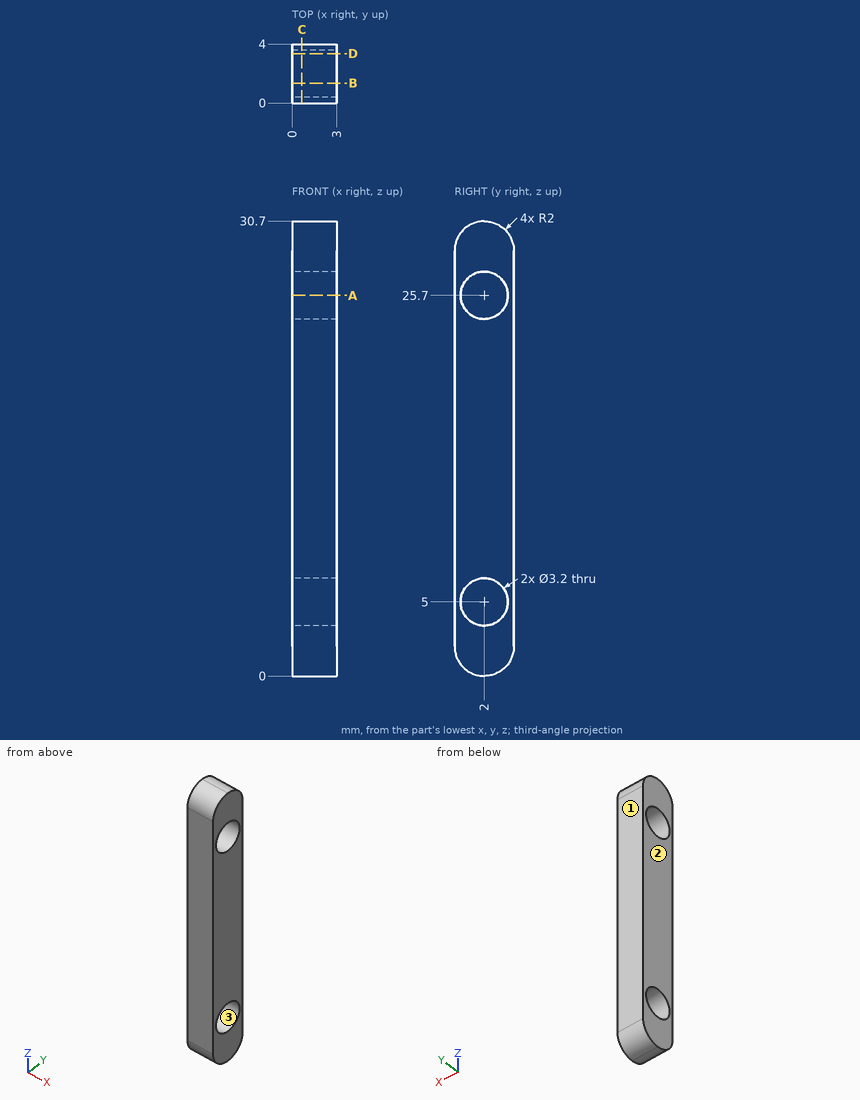
The figure shows three views and two pictorial views of one solid part (mm, origin at its lowest corner). Answer the questions. Round coordinates to 2 decimals unless told otherwise and drop trailing zeros. Write each loop counter-clockwise with the first axis right and the second up, starting at its lowest first coordinate (ties: lowest second). Pieces come first, ordered by that corner, then holes. Notation, with made-up numbers: (2, -2.5) -> (7, -2.5) arc R19 ccw to (7, 22.5) -> close; hole circle Ø1 at (51, 23). An arc over 180 degrees is marked (long way). Answer as a JSON object with one key per item and string values. Group by question number.
Q1. Section D-D (y = 3.35) is taken. Write down the section's boundary in (x, z) (1 decimal).
Q2. Section A-A (z = 25.7) is taken. Write down the section's boundary in (x, y).
Q3. Section C-C (x = 0.65) is taken. Count the separate pieces of the cut face and the enclosed holes in it, plus the area to 3 significant figures.
Q4. Straight lines are drawn through the part: line 1 along Z through (x, y) = (1.35, 2); line 2 along Y through (x, z) = (1.1, 25.7); line 3 along Z through (x, y) = (0.95, 2.95) (1 decimal). For each, find the intervals that lie inside material, in ascending order.
Q5. Section B-B (y = 1.35) is taken. Write down the section's boundary in (x, z).
Q6. Determine the mould class of the marked faces 1, 2 and 3 for opening direction Y: pulls with the +Y half, pulls with the -Y half, needs draft (parallel to the pull), parting line crosses it, or undercut.
Check values:
{
 "1": {"outline": "(0, 0.5) -> (3, 0.5) -> (3, 4.1) -> (0, 4.1) -> close; (0, 5.9) -> (3, 5.9) -> (3, 24.8) -> (0, 24.8) -> close; (0, 26.6) -> (3, 26.6) -> (3, 30.2) -> (0, 30.2) -> close"},
 "2": {"outline": "(0, 0) -> (3, 0) -> (3, 0.4) -> (0, 0.4) -> close; (0, 3.6) -> (3, 3.6) -> (3, 4) -> (0, 4) -> close"},
 "3": {"separate pieces": "1", "enclosed holes": "2", "area": "103 mm^2"},
 "4": {"line 1": "0 to 3.4, 6.6 to 24.1, 27.3 to 30.7", "line 2": "0 to 0.4, 3.6 to 4", "line 3": "0.2 to 3.7, 6.3 to 24.4, 27 to 30.5"},
 "5": {"outline": "(0, 0.11) -> (3, 0.11) -> (3, 3.54) -> (0, 3.54) -> close; (0, 6.46) -> (3, 6.46) -> (3, 24.24) -> (0, 24.24) -> close; (0, 27.16) -> (3, 27.16) -> (3, 30.59) -> (0, 30.59) -> close"},
 "6": {"face 1": "pulls with the +Y half", "face 2": "needs draft", "face 3": "undercut"}
}
